The figure shows three views and two pictorial views of one solid part (mm, origin at its lowest corner). Answer the questions. A direction names the side the tool comes from. Coordinates: 2 decimals unless noted, no trailing zeros. Write each loop counter-clockwise with the first axis right and the second up, starting at its lowest first coordinate (ties: lowest second). Pieces come first, ordered by that corner, then holes.
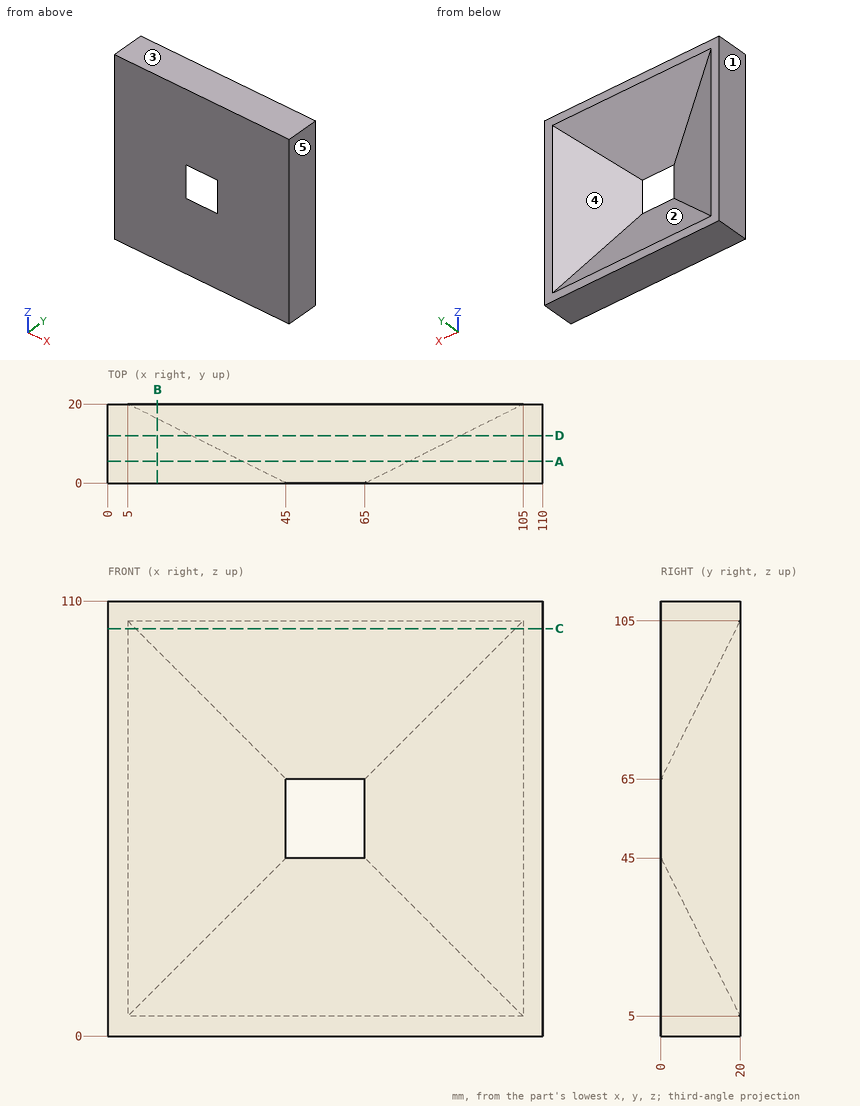
Q1. Given pin 1 (8 mm diameter, centred on x = 11.5, y = 5.5, fed in from -Z); pin 2 (10 mm diameter, centred on x = 57.5, z = 92, fed in from +Y), each flat-ended and moving along its own axis, determine where each tip first touches the part or whether it passes through.
Answers below:
pin 1: stops at z = 0
pin 2: stops at y = 16
Q2. The part is cut by section D-D, the plane y = 12. Write down the section's boundary in (x, z).
Answers below:
outline: (0, 0) - (110, 0) - (110, 110) - (0, 110) - close; hole (21, 21) - (89, 21) - (89, 89) - (21, 89) - close
Q3. Which of the six approach directions +Z, -Z, +X, -X, +Y, -Y give full straight-line access (tool end or side, diameter ignored) to the marked faces 4 and 5?
Answers below:
face 4: +Y
face 5: +Z, -Z, +X, +Y, -Y
Q4. The part is cut by section A-A, the plane y = 5.5. Write down the section's boundary in (x, z).
Answers below:
outline: (0, 0) - (110, 0) - (110, 110) - (0, 110) - close; hole (34, 34) - (76, 34) - (76, 76) - (34, 76) - close
Q5. Find the intervals of material crossed by probe 1 along X at (y, z) = (12.5, 68.5); probe 2 along X at (y, z) = (11.5, 57); probe 3 along Z at (x, y) = (69, 8), in increasing order.
Answers below:
probe 1: x = 0 to 20, 90 to 110
probe 2: x = 0 to 22, 88 to 110
probe 3: z = 0 to 29, 81 to 110
Q6. Determine the mould class of the marked faces 1, 2 and 3 for opening direction Z: released by +Z, released by -Z, zero draft, split by the parting line, or undercut.
Answers below:
face 1: zero draft
face 2: undercut
face 3: released by +Z
Q7. The part is cut by section B-B, the plane x = 12.5. Write down the section's boundary in (y, z).
Answers below:
outline: (0, 0) - (20, 0) - (20, 5) - (16.25, 12.5) - (16.25, 97.5) - (20, 105) - (20, 110) - (0, 110) - close
Q8. The part is cut by section C-C, the plane z = 103. Write down the section's boundary in (x, y), then the cut area to 3 significant figures.
Answers below:
outline: (0, 0) - (110, 0) - (110, 20) - (105, 20) - (103, 19) - (7, 19) - (5, 20) - (0, 20) - close
area: 2,100 mm2
